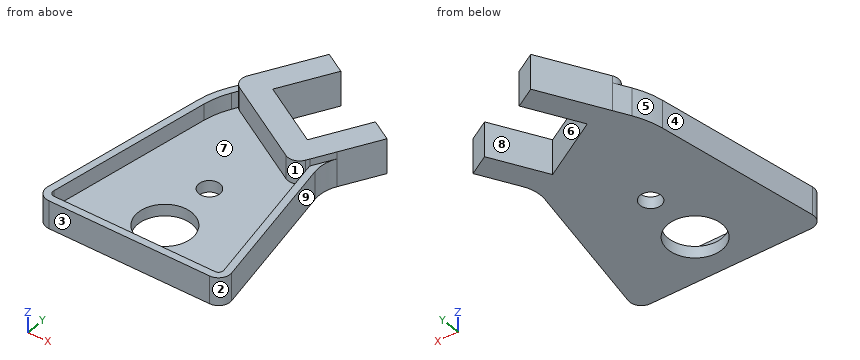
from build123d import *

# Parameters (mm, degrees)
BOSS_EXTRUDE1_DEPTH = 12
SKETCH1_3_R         = 11.5
SKETCH1_3_R_2       = 4.5
BOSS_EXTRUDE2_DEPTH = 5
BOSS_EXTRUDE3_DEPTH = 15


with BuildPart() as part:
    # Sketch1 → Boss-Extrude1 (new body)
    with BuildSketch(Plane.XY):
        with BuildLine():
            ThreePointArc((-38.965270802, 5.868240888), (-37.871454253, 1.786061952), (-34.041232037, 0))
            Line((-34.041232037, 0), (34.041232037, 0))
            ThreePointArc((34.041232037, 0), (37.871454253, 1.786061952), (38.965270802, 5.868240888))
            Line((38.965270802, 5.868240888), (28.21296165, 66.847616303))
            ThreePointArc((28.21296165, 66.847616303), (28.21296165, 72.057061633), (29.994696888, 76.952338968))
            Line((29.994696888, 76.952338968), (25.019759703, 68.335494998))
            ThreePointArc((25.019759703, 68.335494998), (25.11090605, 67.327726281), (25.258538391, 66.32667177))
            Line((25.258538391, 66.32667177), (36.010847543, 5.347296355))
            ThreePointArc((36.010847543, 5.347296355), (35.573320923, 3.714424781), (34.041232037, 3))
            Line((34.041232037, 3), (-34.041232037, 3))
            ThreePointArc((-34.041232037, 3), (-35.573320923, 3.714424781), (-36.010847543, 5.347296355))
            Line((-36.010847543, 5.347296355), (-23.972860012, 73.618116188))
            ThreePointArc((-23.972860012, 73.618116188), (-22.52917578, 79.006019089), (-20.171824836, 84.061374502))
            Line((-20.171824836, 84.061374502), (-18.843846731, 86.361500052))
            ThreePointArc((-18.843846731, 86.361500052), (-19.812658656, 89.05006884), (-19.150635095, 91.830127019))
            Line((-19.150635095, 91.830127019), (-22.769901048, 85.561374502))
            ThreePointArc((-22.769901048, 85.561374502), (-25.348253643, 80.032079519), (-26.927283271, 74.139060721))
            Line((-26.927283271, 74.139060721), (-38.965270802, 5.868240888))
        make_face()
    extrude(amount=BOSS_EXTRUDE1_DEPTH)

    # Sketch1<3> → Boss-Extrude2 (add)
    with BuildSketch(Plane.XY):
        with BuildLine():
            ThreePointArc((25.258538391, 66.32667177), (25.11090605, 67.327726281), (25.019759703, 68.335494998))
            Line((25.019759703, 68.335494998), (24.150635095, 66.830127019))
            ThreePointArc((24.150635095, 66.830127019), (21.114603301, 64.500497887), (17.320508076, 65))
            Line((17.320508076, 65), (-17.320508076, 85))
            ThreePointArc((-17.320508076, 85), (-18.152460566, 85.602112454), (-18.843846731, 86.361500052))
            Line((-18.843846731, 86.361500052), (-20.171824836, 84.061374502))
            ThreePointArc((-20.171824836, 84.061374502), (-22.52917578, 79.006019089), (-23.972860012, 73.618116188))
            Line((-23.972860012, 73.618116188), (-36.010847543, 5.347296355))
            ThreePointArc((-36.010847543, 5.347296355), (-35.573320923, 3.714424781), (-34.041232037, 3))
            Line((-34.041232037, 3), (34.041232037, 3))
            ThreePointArc((34.041232037, 3), (35.573320923, 3.714424781), (36.010847543, 5.347296355))
            Line((36.010847543, 5.347296355), (25.258538391, 66.32667177))
        make_face()
        with Locations((0, 20)):
            Circle(SKETCH1_3_R, mode=Mode.SUBTRACT)
        with Locations((0, 45)):
            Circle(SKETCH1_3_R_2, mode=Mode.SUBTRACT)
    extrude(amount=BOSS_EXTRUDE2_DEPTH)

    # Sketch1<4> → Boss-Extrude3 (add)
    with BuildSketch(Plane.XY):
        with BuildLine():
            Line((25.019759703, 68.335494998), (29.994696888, 76.952338968))
            Line((29.994696888, 76.952338968), (39.150635095, 92.810889132))
            Line((39.150635095, 92.810889132), (30.490381057, 97.810889132))
            Line((30.490381057, 97.810889132), (17.990381057, 76.160254038))
            Line((17.990381057, 76.160254038), (-7.990381057, 91.160254038))
            Line((-7.990381057, 91.160254038), (4.509618943, 112.810889132))
            Line((4.509618943, 112.810889132), (-4.150635095, 117.810889132))
            Line((-4.150635095, 117.810889132), (-19.150635095, 91.830127019))
            ThreePointArc((-19.150635095, 91.830127019), (-19.812658656, 89.05006884), (-18.843846731, 86.361500052))
            ThreePointArc((-18.843846731, 86.361500052), (-18.152460566, 85.602112454), (-17.320508076, 85))
            Line((-17.320508076, 85), (17.320508076, 65))
            ThreePointArc((17.320508076, 65), (21.114603301, 64.500497887), (24.150635095, 66.830127019))
            Line((24.150635095, 66.830127019), (25.019759703, 68.335494998))
        make_face()
    extrude(amount=BOSS_EXTRUDE3_DEPTH)


solid = part.part
Verification items for the finished model (mm, model axes). Face numbers are marked on the shaded views. A direction names the side the tool comes from. Give positions to 0.01 mm unless a question says otherwise; leave off trailing zeros. Order: outer loops, then holes, each group sorted by start corner. A loop starts at its lowest first (then second) coordinate and runs counter-clockwise, first axis right, second up. Notation, with made-up numbers: M 41,29.5 L 90,29.5 A22 cw 90,43.5 Z; hole C 34,13 d6. An arc over 180 degrees is marked long. Use one line per item in the form item = value. Start each with the question number.
Q1. Section check B-B (x = 0). Enter the section's corners in (y, z).
Q2. Section check C-C (z = 7.75). Enter the section's corners in (x, y).
Q3. Mould release check, pull along X, two halves, no side actions. Record for the marked faces 1, 2, 3 and 4: +X half, -X half, draft (parallel to the pull), parting line (faces both ways), or undercut.
Q4. Go/stop test with flat-tipped pins: pin 1 Ø4 at (x, z) = (17.5, 11.5) entering from +Y (3 decimals); pin 2 Ø4 at (y, z) = (56.5, 11) entering from +X; pin 3 Ø3 at (y, z) = (65, 8) entering from +X. Record where each tip stops, or that it passes through.
Q5. Section check D-D (x = 13.5). Enter the section's corners in (y, z).
Q6. Scan lines: line 1 along X through (y, z) = (86, 7.75); line 2 along Y through (x, z) = (0, 3.25); line 3 along X through (y, z) = (68, 5.5). Record each from-to range of solid material in increasing order. Write a range as [from, to].
Q7. Access from +Z, -Z, +X, -X, +Y, -Y to the whole of each face (thin tool, end or side, straight path). Record for the marked faces 5, 6, 7, 8 and 9.
Q8. Section check A-A (y = 45). Enter the section's corners in (x, z), then the cut area to 3 significant figures.
Evaluation:
q1.outline = M 0,0 L 8.5,0 L 8.5,5 L 3,5 L 3,12 L 0,12 Z; M 31.5,0 L 40.5,0 L 40.5,5 L 31.5,5 Z; M 49.5,0 L 86.55,0 L 86.55,15 L 75,15 L 75,5 L 49.5,5 Z; M 105,0 L 115.41,0 L 115.41,15 L 105,15 Z
q2.outline = M -38.97,5.87 A5 ccw -34.04,0 L 34.04,0 A5 ccw 38.97,5.87 L 28.21,66.85 A15 cw 29.99,76.95 L 39.15,92.81 L 30.49,97.81 L 17.99,76.16 L -7.99,91.16 L 4.51,112.81 L -4.15,117.81 L -22.77,85.56 A35 ccw -26.93,74.14 Z; hole M -36.01,5.35 A2 ccw -34.04,3 L 34.04,3 A2 ccw 36.01,5.35 L 25.26,66.33 A18 cw 25.02,68.34 L 24.15,66.83 A5 cw 17.32,65 L -17.32,85 A5 cw -18.84,86.36 L -20.17,84.06 A32 ccw -23.97,73.62 Z
q3.face_1 = undercut
q3.face_2 = +X half
q3.face_3 = draft
q3.face_4 = -X half
q4.pin_1 = 78.775
q4.pin_2 = 30.39
q4.pin_3 = 28.8
q5.outline = M 0,0 L 78.75,0 L 78.75,15 L 67.21,15 L 67.21,5 L 3,5 L 3,12 L 0,12 Z
q6.line_1 = [-22.52, -19.05], [-18.55, 0.95], [23.67, 35.22]
q6.line_2 = [0, 8.5], [31.5, 40.5], [49.5, 86.55], [105, 115.41]
q6.line_3 = [-28.01, -24.96], [12.12, 24.83], [25.04, 28.06]
q7.face_5 = +Z, -Z, -X, +Y
q7.face_6 = +Z, -Z
q7.face_7 = +Z
q7.face_8 = +Z, -Z, +Y
q7.face_9 = +Z, -Z, +X
q8.outline = M -32.07,0 L -4.5,0 L -4.5,5 L -29.02,5 L -29.02,12 L -32.07,12 Z; M 4.5,0 L 32.07,0 L 32.07,12 L 29.02,12 L 29.02,5 L 4.5,5 Z
q8.area = 318 mm2
